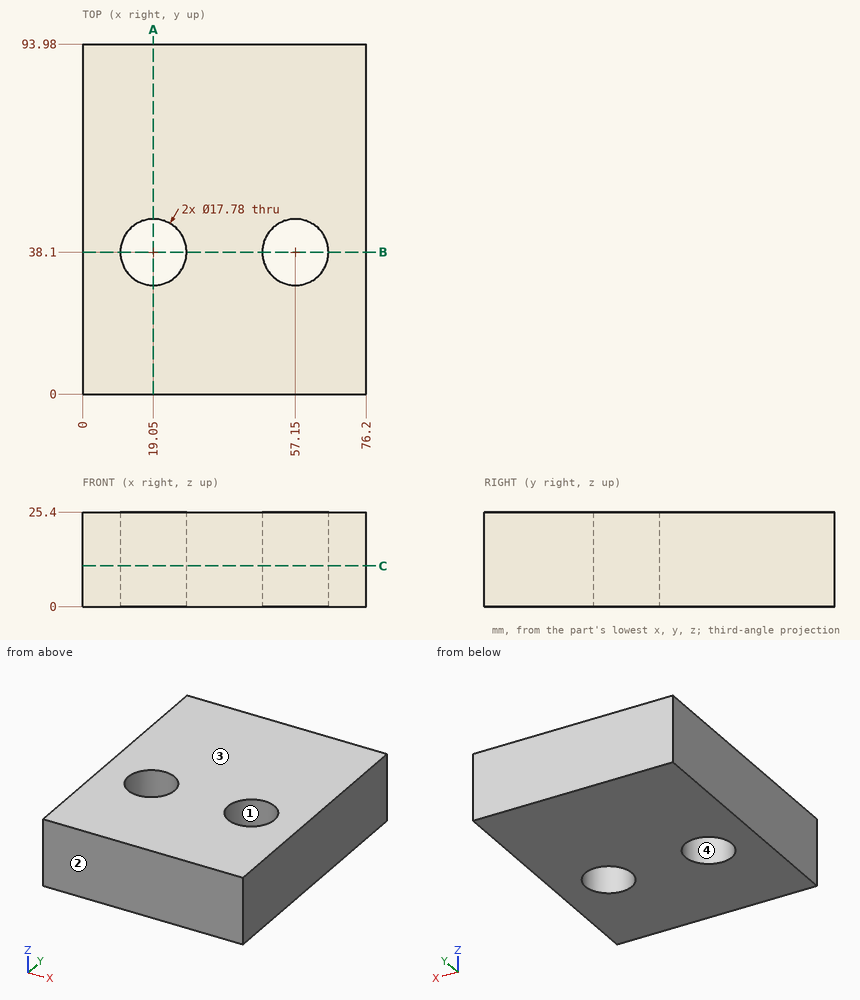
Geometry check sheet. Reference: drawing and pictorial views, mm from the part's lowest x, y, z. Give positions to 0.01 mm unless a question says otherwise; leave off trailing zeros. Order: outer loops, then holes, each group sorted by start corner. A loop starts at its lowest first (then second) coordinate and runs counter-clockwise, first axis right, second up.
1. Section check C-C, the plane z = 11. Enter the section's corners in (x, y), and give its area (3 significant figures).
2. Release check for a two-part mould opening along Y. For the marked faces 1, 2, 3 and 4 record: pulls with the +Y half, pulls with the -Y half, needs draft (parallel to the pull), parting line crosses it, or undercut.
3. Thickness scan on L1, parallel to Y at x = 19.05, z = 18.75; L2, parallel to X at y = 37, z = 19.75; L3, parallel to Y at x = 65, z = 21. Record the ranges inside material, lowest first.
4. Section check A-A, the plane x = 19.05. Enter the section's corners in (y, z).
5. Gauge pin test, flat end, axial feed: pin 1 Ø10.5 at (x, y) = (19.05, 38.1) entering from -Z. Record the tip position at first contact, or that the pin passes through.
6. Section check B-B, the plane y = 38.1. Enter the section's corners in (x, z).
Values follow:
1. outline: (0, 0) - (76.2, 0) - (76.2, 93.98) - (0, 93.98) - close; hole circle Ø17.78 at (19.05, 38.1); hole circle Ø17.78 at (57.15, 38.1)
1. area: 6,660 mm2
2. face 1: undercut
2. face 2: pulls with the -Y half
2. face 3: needs draft
2. face 4: undercut
3. L1: y = 0 to 29.21, 46.99 to 93.98
3. L2: x = 0 to 10.23, 27.87 to 48.33, 65.97 to 76.2
3. L3: y = 0 to 33.93, 42.27 to 93.98
4. outline: (0, 0) - (29.21, 0) - (29.21, 25.4) - (0, 25.4) - close; (46.99, 0) - (93.98, 0) - (93.98, 25.4) - (46.99, 25.4) - close
5. pin 1: passes through
6. outline: (0, 0) - (10.16, 0) - (10.16, 25.4) - (0, 25.4) - close; (27.94, 0) - (48.26, 0) - (48.26, 25.4) - (27.94, 25.4) - close; (66.04, 0) - (76.2, 0) - (76.2, 25.4) - (66.04, 25.4) - close
